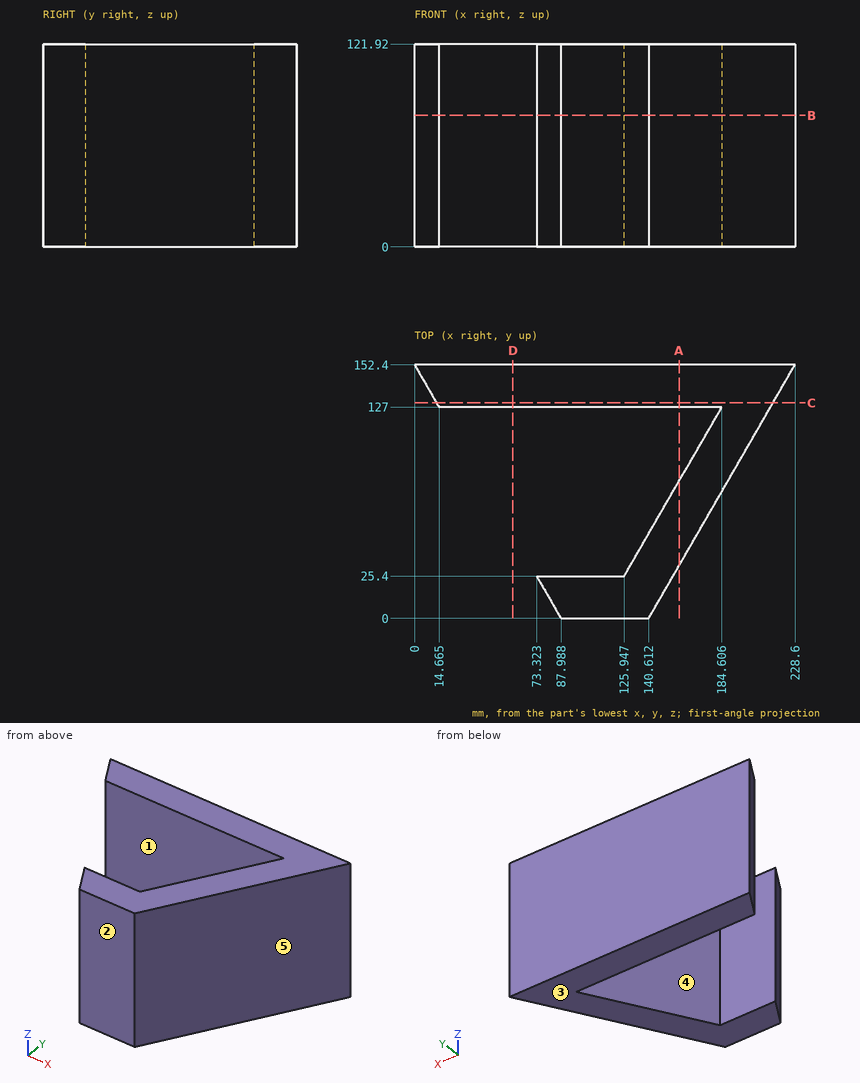
Geometry check sheet. Reference: drawing and pictorial views, mm from the part's lowest x, y, z. A direction names the side the tool comes from. Coordinates: 2 decimals unless noted, no trailing zeros. Write each loop counter-clockwise with the first axis right and the second up, starting at its lowest first coordinate (ties: lowest second). Pieces come first, ordered by that corner, then holes.
Item 1: Cross-section at D-D on x = 59. Record the boundary of the cut face in (y, z).
Numbers:
outline: (127, 0) - (152.4, 0) - (152.4, 121.92) - (127, 121.92) - close
Item 2: Depth check by flat-ended pin: pin 1 Ø6 at (y, z) = (66, 89.5) entering from -X (1 decimal); pin 2 Ø12 at (y, z) = (133.5, 66) entering from -X; pin 3 Ø1 at (y, z) = (25.5, 70) entering from -X. Enter the tip coordinate at first touch or a pass-through.
Numbers:
pin 1: stops at x = 147.7
pin 2: stops at x = 7.45
pin 3: stops at x = 73.32
Item 3: Cross-section at B-B on z = 79. Record the boundary of the cut face in (x, y) (1 decimal).
Numbers:
outline: (0, 152.4) - (14.7, 127) - (184.6, 127) - (125.9, 25.4) - (73.3, 25.4) - (88, 0) - (140.6, 0) - (228.6, 152.4) - close
Item 4: Cross-section at C-C on y = 129.5. Record the boundary of the cut face in (x, z), then the cut area to 3 significant figures.
Numbers:
outline: (13.22, 0) - (215.38, 0) - (215.38, 121.92) - (13.22, 121.92) - close
area: 24,600 mm2
Item 5: Mould release check, pull along Y, two halves, no side actions. Record for the marked faces 1, 2 and 3: released by +Y, released by -Y, zero draft, split by the parting line, or undercut.
Numbers:
face 1: undercut
face 2: released by -Y
face 3: zero draft
Item 6: Cross-section at A-A on x = 159. Record the boundary of the cut face in (y, z), then the cut area to 3 significant figures.
Numbers:
outline: (31.85, 0) - (82.65, 0) - (82.65, 121.92) - (31.85, 121.92) - close; (127, 0) - (152.4, 0) - (152.4, 121.92) - (127, 121.92) - close
area: 9,290 mm2
Item 7: Scan lines: probe 1 along Y at (x, z) = (16, 88.5); probe 2 along Y at (x, z) = (128, 87) (1 decimal); probe 3 along Y at (x, z) = (155.5, 17) (1 decimal). Record each from-to range of solid material in increasing order.
Numbers:
probe 1: y = 127 to 152.4
probe 2: y = 0 to 29, 127 to 152.4
probe 3: y = 25.8 to 76.6, 127 to 152.4
Item 8: Access from +Z, -Z, +X, -X, +Y, -Y to the whole of each face (thin tool, end or side, straight path). Record for the marked faces 4 and 5.
Numbers:
face 4: +Z, -Z, -X
face 5: +Z, -Z, +X, -Y
